Autodesk Inventor part; units mm, degrees
ref_plane "作業平面2" through (4, 0, 0) normal (1, 0, 0) x (0, 1, 0)
ref_plane "YZ Plane" through (0, 0, 0) normal (1, 0, 0) x (0, 1, 0)
ref_plane "XZ Plane" through (0, 0, 0) normal (0, 1, 0) x (-1, 0, 0)
sketch "スケッチ1" plane through (0, 0, 0) normal (0, 1, 0) x (-1, 0, 0)
  circle A0 centre (0, 0) radius 5
  dimension "d0" = 10
extrude "押し出し1" add sketch "スケッチ1" along normal blind 27.8
sketch "スケッチ2" plane through (0, 27.8, 0) normal (0, 1, 0) x (1, 0, 0)
  circle A0 centre (0, 0) radius 4
  dimension "d3" = 8
extrude "押し出し2" add sketch "スケッチ2" along normal blind 41
sketch "スケッチ3" plane through (0, 68.8, 0) normal (0, 1, 0) x (1, 0, 0)
  circle A0 centre (0, 0) radius 3
  dimension "d6" = 6
extrude "押し出し3" [suppressed]
sketch "スケッチ4" plane through (0, 0, 0) normal (0, -1, 0) x (1, 0, 0)
  circle A0 centre (0, 0) radius 4
  circle A1 centre (0, 0) radius 4
  dimension "d9" = 8
extrude "押し出し4" add sketch "スケッチ4" along normal blind 31
sketch "スケッチ5" plane through (0, -31, 0) normal (0, -1, 0) x (1, 0, 0)
  circle A0 centre (0, 0) radius 4
  circle A1 centre (0, 0) radius 3
  dimension "d12" = 6
extrude "押し出し5" add sketch "スケッチ5" along normal blind 17 contours A1
sketch "スケッチ6" plane through (0, 0, 0) normal (0, -1, 0) x (1, 0, 0)
  circle A0 centre (0, 0) radius 5
  point P0 (5, 0)
ref_plane "作業平面1" through (5, 0, 0) normal (1, 0, 0) x (0, 1, 0)
sketch "スケッチ7" plane through (5, 0, 0) normal (1, 0, 0) x (0, 1, 0)
  line L0 (4.4, 1.5) -> (24.4, 1.5)
  line L1 (24.4, 1.5) -> (24.4, -1.5)
  line L2 (24.4, -1.5) -> (4.4, -1.5)
  line L3 (4.4, -1.5) -> (4.4, 1.5)
  line L4 (4.4, 1.5) -> (24.4, -1.5) construction
  line L5 (24.4, 1.5) -> (4.4, -1.5) construction
  line L6 (0, -5) -> (0, 5)
  point P0 (0, 0)
  point P1 (14.4, 0)
  dimension "d15" = 20
  dimension "d16" = 3
  dimension "d17" = 4.4
extrude "押し出し6" cut sketch "スケッチ7" against normal blind 1.8
sketch "スケッチ8" plane through (5, 0, 0) normal (1, 0, 0) x (0, 1, 0)
  point P0 (0, 0)
sketch "スケッチ9" plane through (5, 0, 0) normal (1, 0, 0) x (0, 1, 0)
  point P0 (0, 0)
ref_plane "作業平面2" through (4, 0, 0) normal (1, 0, 0) x (0, 1, 0)
sketch "スケッチ10" plane through (4, 0, 0) normal (1, 0, 0) x (0, 1, 0)
  line L0 (49.8, 1.5) -> (65.8, 1.5)
  line L1 (65.8, 1.5) -> (65.8, -1.5)
  line L2 (65.8, -1.5) -> (49.8, -1.5)
  line L3 (49.8, -1.5) -> (49.8, 1.5)
  line L4 (49.8, 1.5) -> (65.8, -1.5) construction
  line L5 (65.8, 1.5) -> (49.8, -1.5) construction
  line L6 (-31, 1.5) -> (-15, 1.5)
  line L7 (-15, 1.5) -> (-15, -1.5)
  line L8 (-15, -1.5) -> (-31, -1.5)
  line L9 (-31, -1.5) -> (-31, 1.5)
  line L10 (-31, 1.5) -> (-15, -1.5) construction
  line L11 (-15, 1.5) -> (-31, -1.5) construction
  line L12 (-31, 4) -> (-31, -4)
  line L13 (68.8, -4) -> (68.8, 4)
  point P0 (0, 0)
  point P1 (57.8, 0)
  point P2 (-23, 0)
  dimension "d21" = 16
  dimension "d22" = 3
  dimension "d23" = 16
  dimension "d24" = 3
  dimension "d25" = 0
  dimension "d26" = 3
extrude "押し出し8" cut sketch "スケッチ10" against normal blind 1.8
properties part number "shoulder1_shaft" material "鋼、炭素鋼"
Can you work these out from the model? Positions are in its coordinate system, mm. A direction names the side the tool comes from. Coordinates: 2 decimals unless noted, no trailing zeros. Order: outer loops, then holes, each group sorted by start corner. A loop starts at its lowest first (then second) coordinate and runs counter-clockwise, first axis right, second up. Notation, with made-up numbers: (-39.5, 15) - (-13.5, 15) arc R35 ccw to (-13.5, 49) - close; hole circle Ø7 at (-14.5, 25). An arc over 180 degrees is marked (long way). Answer as a JSON object with one key per item and string values. Group by question number.
Q1. Imagine slicing it at C-C (y = -34). Please give me the cut outline in (x, z), and give its area (3 significant figures).
Q2. Imagine slicing it at B-B (x = 0). Please give me the cut outline in (y, z).
Q3. Will these pins go through, and if not, where does the flat tip stop? P1, Ø1.3, axis at x = 4.5, y = 10.5, coming from the -Z side; P2, Ø2.5, axis at y = 60, z = 0.5, coming from the +X side; P3, Ø5, axis at y = -7, z = 3.5, coming from the +X side.
Q4. We'd pull the mould along Y, two halves only. Please class faces 1 (the face through (3, 65.8, 0)), 2 (the face through (0, -48, 0)), 3 (the face through (-3.2, -15.3, 2.4)), 4 (the face through (3, 49.8, 0)): +Y half, -Y half, draft (parallel to the pull), parting line (faces both ways), or undercut.
Q5. On a 3-axis mill with a long thin cutter (end or side, diameter ignored), from which of +Z, -Z, +X, -X, +Y, -Y can I reach the whole of each face in a straight line? I mean faces 5 (the face through (-3.2, 48, -2.4)), 6 (the face through (0, 68.8, 0)), 7 (the face through (-4.77, 13.71, -1.5)), 8 (the face through (3, -15, 0)), 9 (the face through (-3, -39, 0)). Say none if no direction works.
Q6. I need wall thicknesses on line 1 (Y direction, x = 2.5, z = -0.5); line 2 (Z direction, x = -0.25, y = 12.5); line 3 (Z direction, x = 3, y = 21). Which ranges of each line are inside material? Lowest first, please. Write a range as from..to.
Q7. Imagine slicing it at A-A (z = 0). Please give me the cut outline in (x, y), and give its area (3 significant figures).
Determined:
{
 "1": {"outline": "circle Ø6 at (0, 0)", "area": "28.3 mm2"},
 "2": {"outline": "(-48, -3) - (-31, -3) - (-31, -4) - (0, -4) - (0, -5) - (27.8, -5) - (27.8, -4) - (68.8, -4) - (68.8, 4) - (27.8, 4) - (27.8, 5) - (0, 5) - (0, 4) - (-31, 4) - (-31, 3) - (-48, 3) - close"},
 "3": {"P1": "stops at z = -3.19", "P2": "stops at x = 3.71", "P3": "stops at x = 3.87"},
 "4": {"face 1": "undercut", "face 2": "-Y half", "face 3": "draft", "face 4": "undercut"},
 "5": {"face 5": "+Y", "face 6": "+Z, -Z, +X, -X, +Y", "face 7": "+Y, -Y", "face 8": "+X", "face 9": "-Y"},
 "6": {"line 1": "y = -48..-31, -15..49.8, 65.8..68.8", "line 2": "z = -4.99..4.99", "line 3": "z = -4..4"},
 "7": {"outline": "(-5, 0) - (-4, 0) - (-4, -31) - (-3, -31) - (-3, -48) - (3, -48) - (3, -31) - (2.2, -31) - (2.2, -15) - (4, -15) - (4, 0) - (5, 0) - (5, 4.4) - (3.2, 4.4) - (3.2, 24.4) - (5, 24.4) - (5, 27.8) - (4, 27.8) - (4, 49.8) - (2.2, 49.8) - (2.2, 65.8) - (4, 65.8) - (4, 68.8) - (-4, 68.8) - (-4, 27.8) - (-5, 27.8) - close", "area": "862 mm2"}
}
